Verification items for this drawing (mm, ordinates from the low corner). A direction names the side the tool comes from. Round coordinates to 2 decimals unless told otherwise and drop trailing zeros. Loops run counter-clockwise (first coordinate to the right, second up) from the corner with the lowest first, then second, coordinate; pieces in that order, holes last. Notation, with made-up numbers: (56.25, -16.75) -> (90.25, -16.75) arc R27 cw to (90.25, 16.25) -> close; hole circle Ø5 at (11.5, 62.5). An arc over 180 degrees is marked (long way). Use a Markdown table: item, result. Add a question column.
Q1. Release check for a two-part mould opening along Z. For the marked faces 1, 2 and 3 record: released by +Z, released by -Z, zero draft, split by the parting line, or undercut.
Q2. Set-up check for the marked faces 4 and 5: record each of +Z, -Z, +X, -X, +Y, -Y from which the full face is reachable in a straight line by a thin tool's end or side.
Q3. Sectioned sample at D-D, the plane y = 3. Enter the section's corners in (x, z).
Q4. Material ranges on L1, parallel to Y at x = 11, z = 27 (1 decimal); L2, parallel to X at y = 4.5, z = 13 (1 decimal); L3, parallel to Z at x = 13.5, y = 25 (1 decimal), recorded low to high.
Q5. Gauge pin test, flat ends, axial feed: P1, Ø6, axis at x = 17, y = 16.5, coming from the +Z side (3 decimals); P2, Ø10, axis at y = 19, z = 18.5, coming from the +X side (3 decimals); P3, Ø1.5, axis at x = 11, y = 8, coming from the -Z side; P4, Ø2, axis at x = 31.5, z = 12, coming from the +Y side. Record the tip position at first contact, or that the pin passes through.
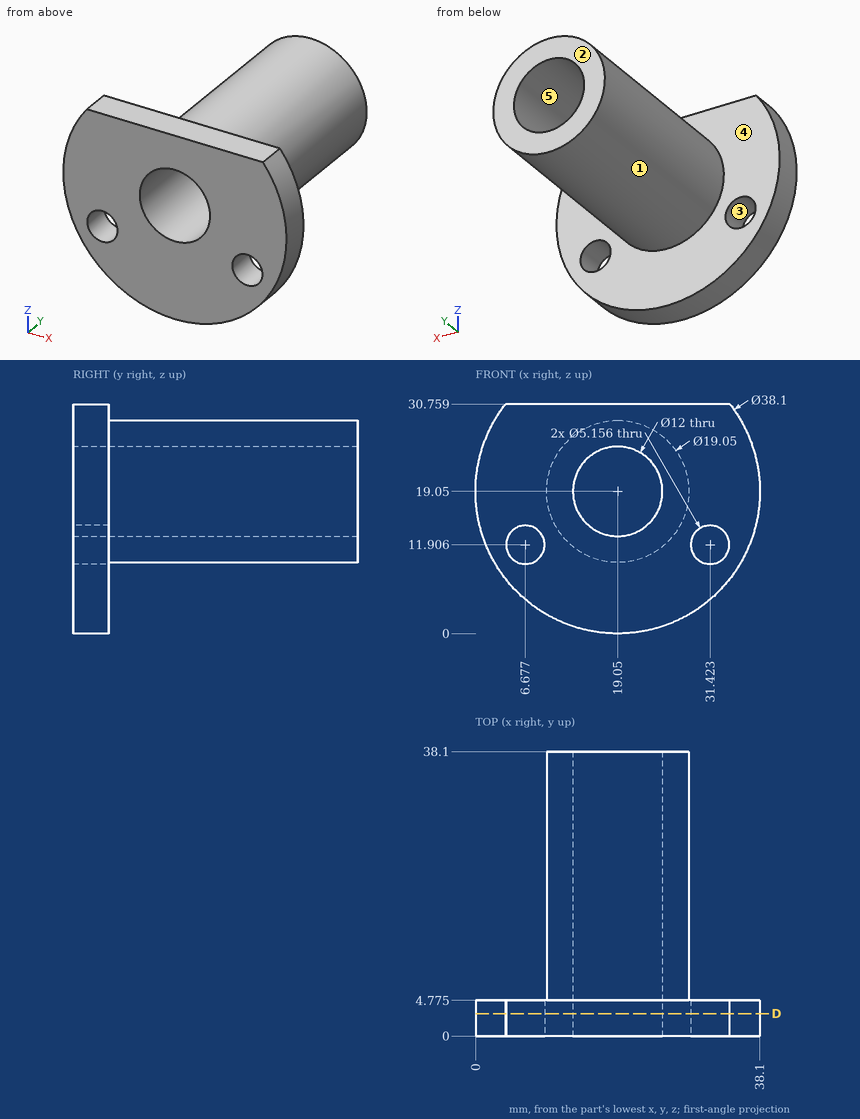
Values:
| question | item | result |
|---|---|---|
| 1 | face 1 | split by the parting line |
| 1 | face 2 | zero draft |
| 1 | face 3 | undercut |
| 2 | face 4 | +Y |
| 2 | face 5 | +Y, -Y |
| 3 | outline | (4.02, 30.76) arc R19.05 ccw (long way) to (34.08, 30.76) -> close; hole circle Ø5.16 at (6.68, 11.91); hole circle Ø12 at (19.05, 19.05); hole circle Ø5.16 at (31.42, 11.91) |
| 4 | L1 | 0 to 4.8 |
| 4 | L2 | 1 to 4.3, 9 to 29.1, 33.8 to 37.1 |
| 4 | L3 | 11.3 to 16.8, 21.3 to 26.8 |
| 5 | P1 | z = 28.575 |
| 5 | P2 | x = 28.575 |
| 5 | P3 | z = 12.93 |
| 5 | P4 | through |
